Work out the finished part from the listing and answer in its coordinate system (mm). Give positions to 0.01 mm unless a question says otherwise; leave off trailing zeros. Loops run counter-clockwise (first coordinate to the right, second up) from the corner with the lowest first, then second, coordinate; pieces in that order, holes last. Notation, with made-up numbers: (0, -6) - (30, -6) arc R14 ccw to (30, 16) - close; hole circle Ø4 at (64.5, 86.5). An arc over 180 degrees is marked (long way). One line per question, with ' | ' between items. Start each with the question number.
1. Section C-C (x = 15) is taken. Determine the outline of the cut face in (y, z).
2. Section B-B (y = 59) is taken. Determine the outline of the cut face in (x, z), plus the area to 3 significant figures.
3. Section D-D (x = -9) is taken. Determine the outline of the cut face in (y, z), plus the area to 3 significant figures.
4. For a pull along X with two mould halves and no side action, classify faces 1 (the face through (-1, 7, 3)), 2 (the face through (44.396, 22.872, 1.479)), 3 (the face through (0.09, 66.316, 1.479)) as released by +X, released by -X, zero draft, split by the parting line, or undercut.
5. Find the intervals of material crossed by line 1 (X direction, y = 26, z = 2.3); line 2 (Y direction, x = 26, z = 2.8); line 3 (X direction, y = 27.5, z = 2.95), in increasing order.
6. Each of these flat-tipped pins is pushed along its axis until it touches: pin 1 (1.5 mm diameter, centred on y = 49, z = 1, fed in from -X); pin 2 (1.5 mm diameter, centred on y = 42.5, z = 2, fed in from +X). Where does it stop, or does it pass through?
7. Section A-A (z = 2.55) is taken. Give the number of separate pieces and of enclosed holes in the cut face, plus the area to 3 significant figures.
from build123d import *

# Parameters (mm, degrees)
SKETCH1_R           = 4
BOSS_EXTRUDE2_DEPTH = 3


with BuildPart() as part:
    # Sketch1 → Boss-Extrude2 (new body)
    with BuildSketch(Plane.XY):
        with BuildLine():
            Line((-6.012571554, 64.307027075), (-33.069131887, 43.948066126))
            ThreePointArc((-33.069131887, 43.948066126), (2.07e-06, -55), (33.069128578, 43.948068616))
            Line((33.069128578, 43.948068616), (6.012566712, 64.307027528))
            ThreePointArc((6.012566712, 64.307027528), (-2.497e-06, 66.316469598), (-6.012571554, 64.307027075))
        make_face()
        with BuildLine():
            ThreePointArc((-30.698965133, -43.203238849), (-30.703332787, -43.196953768), (-30.701976961, -43.189421147))
            Line((-30.701976961, -43.189421147), (-29.091901743, -40.68182114))
            ThreePointArc((-29.091901743, -40.68182114), (-29.085616662, -40.677453486), (-29.078084041, -40.678809312))
            Line((-29.078084041, -40.678809312), (-24.88753101, -43.369471925))
            ThreePointArc((-24.88753101, -43.369471925), (-24.883163356, -43.375757006), (-24.884519182, -43.383289627))
            Line((-24.884519182, -43.383289627), (-26.4945944, -45.890889633))
            ThreePointArc((-26.4945944, -45.890889633), (-26.500879481, -45.895257287), (-26.508412102, -45.893901462))
            Line((-26.508412102, -45.893901462), (-30.698965133, -43.203238849))
        make_face(mode=Mode.SUBTRACT)
        with BuildLine():
            ThreePointArc((-4.98444277, -52.764580253), (-4.99136781, -52.76132104), (-4.993959941, -52.754119686))
            Line((-4.993959941, -52.754119686), (-4.853393903, -49.777436769))
            ThreePointArc((-4.853393903, -49.777436769), (-4.85013469, -49.770511729), (-4.842933336, -49.767919598))
            Line((-4.842933336, -49.767919598), (0.131523351, -50.002825259))
            ThreePointArc((0.131523351, -50.002825259), (0.138448391, -50.006084472), (0.141040522, -50.013285826))
            Line((0.141040522, -50.013285826), (0.000474484, -52.989968743))
            ThreePointArc((0.000474484, -52.989968743), (-0.002784729, -52.996893783), (-0.009986083, -52.999485914))
            Line((-0.009986083, -52.999485914), (-4.98444277, -52.764580253))
        make_face(mode=Mode.SUBTRACT)
        with BuildLine():
            ThreePointArc((-48.187724044, -22.065613117), (-48.188364003, -22.05798625), (-48.183423512, -22.052140721))
            Line((-48.183423512, -22.052140721), (-45.535257468, -20.685533022))
            ThreePointArc((-45.535257468, -20.685533022), (-45.527630602, -20.684893064), (-45.521785073, -20.689833554))
            Line((-45.521785073, -20.689833554), (-43.237990999, -25.115292245))
            ThreePointArc((-43.237990999, -25.115292245), (-43.23735104, -25.122919112), (-43.242291531, -25.12876464))
            Line((-43.242291531, -25.12876464), (-45.890457575, -26.495372339))
            ThreePointArc((-45.890457575, -26.495372339), (-45.898084441, -26.496012298), (-45.90392997, -26.491071808))
            Line((-45.90392997, -26.491071808), (-48.187724044, -22.065613117))
        make_face(mode=Mode.SUBTRACT)
        with BuildLine():
            ThreePointArc((-52.764620675, 4.984487199), (-52.761361462, 4.991412238), (-52.754160108, 4.994004369))
            Line((-52.754160108, 4.994004369), (-49.777477191, 4.853438332))
            ThreePointArc((-49.777477191, 4.853438332), (-49.770552151, 4.850179119), (-49.76796002, 4.842977765))
            Line((-49.76796002, 4.842977765), (-50.002865681, -0.131478922))
            ThreePointArc((-50.002865681, -0.131478922), (-50.006124893, -0.138403962), (-50.013326248, -0.140996093))
            Line((-50.013326248, -0.140996093), (-52.990009165, -0.000430055))
            ThreePointArc((-52.990009165, -0.000430055), (-52.996934204, 0.002829158), (-52.999526335, 0.010030512))
            Line((-52.999526335, 0.010030512), (-52.764620675, 4.984487199))
        make_face(mode=Mode.SUBTRACT)
        with BuildLine():
            ThreePointArc((22.065657545, -48.187683622), (22.058030679, -48.188323581), (22.05218515, -48.183383091))
            Line((22.05218515, -48.183383091), (20.685577451, -45.535217046))
            ThreePointArc((20.685577451, -45.535217046), (20.684937492, -45.52759018), (20.689877983, -45.521744651))
            Line((20.689877983, -45.521744651), (25.115336674, -43.237950577))
            ThreePointArc((25.115336674, -43.237950577), (25.12296354, -43.237310619), (25.128809069, -43.242251109))
            Line((25.128809069, -43.242251109), (26.495416768, -45.890417153))
            ThreePointArc((26.495416768, -45.890417153), (26.496056726, -45.898044019), (26.491116236, -45.903889548))
            Line((26.491116236, -45.903889548), (22.065657545, -48.187683622))
        make_face(mode=Mode.SUBTRACT)
        with BuildLine():
            ThreePointArc((43.203283277, -30.698924711), (43.196998196, -30.703292365), (43.189465575, -30.701936539))
            Line((43.189465575, -30.701936539), (40.681865569, -29.091861321))
            ThreePointArc((40.681865569, -29.091861321), (40.677497915, -29.08557624), (40.678853741, -29.078043619))
            Line((40.678853741, -29.078043619), (43.369516354, -24.887490588))
            ThreePointArc((43.369516354, -24.887490588), (43.375801435, -24.883122935), (43.383334056, -24.88447876))
            Line((43.383334056, -24.88447876), (45.890934062, -26.494553978))
            ThreePointArc((45.890934062, -26.494553978), (45.895301716, -26.500839059), (45.89394589, -26.508371681))
            Line((45.89394589, -26.508371681), (43.203283277, -30.698924711))
        make_face(mode=Mode.SUBTRACT)
        with BuildLine():
            ThreePointArc((52.990013172, 0.000514906), (52.996938211, -0.002744307), (52.999530342, -0.009945661))
            Line((52.999530342, -0.009945661), (52.764624682, -4.984402348))
            ThreePointArc((52.764624682, -4.984402348), (52.761365469, -4.991327388), (52.754164115, -4.993919519))
            Line((52.754164115, -4.993919519), (49.777481198, -4.853353481))
            ThreePointArc((49.777481198, -4.853353481), (49.770556158, -4.850094268), (49.767964027, -4.842892914))
            Line((49.767964027, -4.842892914), (50.002869687, 0.131563773))
            ThreePointArc((50.002869687, 0.131563773), (50.0061289, 0.138488813), (50.013330254, 0.141080944))
            Line((50.013330254, 0.141080944), (52.990013172, 0.000514906))
        make_face(mode=Mode.SUBTRACT)
        with BuildLine():
            ThreePointArc((-43.203279271, 30.699009562), (-43.19699419, 30.703377216), (-43.189461569, 30.70202139))
            Line((-43.189461569, 30.70202139), (-40.681861562, 29.091946172))
            ThreePointArc((-40.681861562, 29.091946172), (-40.677493908, 29.085661091), (-40.678849734, 29.07812847))
            Line((-40.678849734, 29.07812847), (-43.369512347, 24.887575439))
            ThreePointArc((-43.369512347, 24.887575439), (-43.375797428, 24.883207785), (-43.383330049, 24.884563611))
            Line((-43.383330049, 24.884563611), (-45.890930055, 26.494638829))
            ThreePointArc((-45.890930055, 26.494638829), (-45.895297709, 26.50092391), (-45.893941883, 26.508456531))
            Line((-45.893941883, 26.508456531), (-43.203279271, 30.699009562))
        make_face(mode=Mode.SUBTRACT)
        with BuildLine():
            ThreePointArc((-22.065653538, 48.187768473), (-22.058026672, 48.188408431), (-22.052181143, 48.183467941))
            Line((-22.052181143, 48.183467941), (-20.685573444, 45.535301897))
            ThreePointArc((-20.685573444, 45.535301897), (-20.684933486, 45.52767503), (-20.689873976, 45.521829502))
            Line((-20.689873976, 45.521829502), (-25.115332667, 43.238035428))
            ThreePointArc((-25.115332667, 43.238035428), (-25.122959534, 43.237395469), (-25.128805062, 43.242335959))
            Line((-25.128805062, 43.242335959), (-26.495412761, 45.890502003))
            ThreePointArc((-26.495412761, 45.890502003), (-26.49605272, 45.89812887), (-26.49111223, 45.903974398))
            Line((-26.49111223, 45.903974398), (-22.065653538, 48.187768473))
        make_face(mode=Mode.SUBTRACT)
        with BuildLine():
            ThreePointArc((-0.309437301, 52.998669808), (-0.302221838, 52.996117213), (-0.298924693, 52.989210153))
            Line((-0.298924693, 52.989210153), (-0.14203469, 50.013342964))
            ThreePointArc((-0.14203469, 50.013342964), (-0.144587285, 50.006127501), (-0.151494345, 50.002830356))
            Line((-0.151494345, 50.002830356), (-5.10710915, 49.741566538))
            ThreePointArc((-5.10710915, 49.741566538), (-5.114324612, 49.744119133), (-5.117621758, 49.751026193))
            Line((-5.117621758, 49.751026193), (-5.274511761, 52.726893382))
            ThreePointArc((-5.274511761, 52.726893382), (-5.271959166, 52.734108845), (-5.265052106, 52.73740599))
            Line((-5.265052106, 52.73740599), (-0.309437301, 52.998669808))
        make_face(mode=Mode.SUBTRACT)
        with Locations((0, 59)):
            Circle(SKETCH1_R, mode=Mode.SUBTRACT)
        with BuildLine():
            ThreePointArc((48.187728051, 22.065697967), (48.188368009, 22.0580711), (48.183427519, 22.052225572))
            Line((48.183427519, 22.052225572), (45.535261475, 20.685617873))
            ThreePointArc((45.535261475, 20.685617873), (45.527634608, 20.684977914), (45.52178908, 20.689918404))
            Line((45.52178908, 20.689918404), (43.237995006, 25.115377096))
            ThreePointArc((43.237995006, 25.115377096), (43.237355047, 25.123003962), (43.242295537, 25.128849491))
            Line((43.242295537, 25.128849491), (45.890461581, 26.49545719))
            ThreePointArc((45.890461581, 26.49545719), (45.898088448, 26.496097148), (45.903933977, 26.491156658))
            Line((45.903933977, 26.491156658), (48.187728051, 22.065697967))
        make_face(mode=Mode.SUBTRACT)
        with BuildLine():
            ThreePointArc((4.984446777, 52.764665104), (4.991371816, 52.761405891), (4.993963947, 52.754204537))
            Line((4.993963947, 52.754204537), (4.85339791, 49.77752162))
            ThreePointArc((4.85339791, 49.77752162), (4.850138697, 49.77059658), (4.842937343, 49.768004449))
            Line((4.842937343, 49.768004449), (-0.131519344, 50.002910109))
            ThreePointArc((-0.131519344, 50.002910109), (-0.138444384, 50.006169322), (-0.141036515, 50.013370676))
            Line((-0.141036515, 50.013370676), (-0.000470477, 52.990053593))
            ThreePointArc((-0.000470477, 52.990053593), (0.002788736, 52.996978633), (0.00999009, 52.999570764))
            Line((0.00999009, 52.999570764), (4.984446777, 52.764665104))
        make_face(mode=Mode.SUBTRACT)
        with BuildLine():
            ThreePointArc((30.69896914, 43.203323699), (30.703336794, 43.197038618), (30.701980968, 43.189505997))
            Line((30.701980968, 43.189505997), (29.09190575, 40.681905991))
            ThreePointArc((29.09190575, 40.681905991), (29.085620669, 40.677538337), (29.078088048, 40.678894163))
            Line((29.078088048, 40.678894163), (24.887535017, 43.369556776))
            ThreePointArc((24.887535017, 43.369556776), (24.883167363, 43.375841857), (24.884523189, 43.383374478))
            Line((24.884523189, 43.383374478), (26.494598407, 45.890974484))
            ThreePointArc((26.494598407, 45.890974484), (26.500883488, 45.895342138), (26.508416109, 45.893986312))
            Line((26.508416109, 45.893986312), (30.69896914, 43.203323699))
        make_face(mode=Mode.SUBTRACT)
    extrude(amount=BOSS_EXTRUDE2_DEPTH)


solid = part.part
Conclusion:
1) outline: (-52.92, 0) - (57.54, 0) - (57.54, 3) - (-52.92, 3) - close
2) outline: (-13.07, 0) - (-4, 0) - (-4, 3) - (-13.07, 3) - close; (4, 0) - (13.07, 0) - (13.07, 3) - (4, 3) - close | area: 54.4 mm²
3) outline: (-54.26, 0) - (62.06, 0) - (62.06, 3) - (-54.26, 3) - close | area: 349 mm²
4) face 1: zero draft | face 2: undercut | face 3: split by the parting line
5) line 1: -48.47 to -45.12, -42.66 to 44.93, 46.16 to 48.47 | line 2: -48.47 to -46.16, -44.93 to 42.66, 45.12 to 49.27 | line 3: -47.63 to -45.26, -41.69 to 47.63
6) pin 1: x = -27.35 | pin 2: x = 35.8
7) separate pieces: 1 | enclosed holes: 14 | area: 9,570 mm²
